CAD build for the part. Positions are in the model's coordinates, mm. A direction names the side the tool comes from. Coordinates: 2 decimals unless noted, no trailing zeros. Order: outer loops, then holes, each group sorted by start corner. A loop starts at its lowest first (then second) coordinate and runs counter-clockwise, first axis right, second up. Notation, with made-up numbers: (55.5, 8) - (109.5, 8) arc R26 cw to (109.5, 27) - close; hole circle Ø5 at (68, 0). An arc over 180 degrees is marked (long way). Write each question's results on one line, items separated by ' | '. Start each with the question number.
Q1. Wall check: probe 1 along Y at (x, z) = (2, -4); probe 2 along Z at (x, y) = (4, -3); probe 3 along Z at (x, y) = (-0.5, -10). Give the ranges that are in metal, low to high.
Q2. Band-saw the part on B-B, the plane x = 0. Write the cut outline in (y, z).
Q3. Which spindle directions (+Z, -Z, +X, -X, +Y, -Y) get a long thin tool onto all of the face, cutting with end or side? Do faces 5 (the flat face through (4.5, 0, -18)), 6 (the flat face through (-0.1, 7.934, -35.6)), 7 (the flat face through (0, 17.5, -3)). Say none if no direction does.
Q4. Band-saw the part on D-D, the plane y = -15.5. Write the cut outline in (x, z).
Q5. Pull direction Y, two halves, no side cores. Call faces 1 (the flat face through (0, 0, -35.181)), 2 (the flat face through (-0.063, 18.514, -32.62)), 3 (the flat face through (0, 0, -5.153)), 4 (the flat face through (0, 13, -36)): released by +Y, released by -Y, zero draft, split by the parting line, or undercut.
Q6. Band-saw the part on C-C, the plane y = 0.5. Write the cut outline in (x, z).
Q7. Pin check, flat tips, straight feed: P1, Ø2, axis at x = 1, y = -0.5, coming from the -Z side; P2, Ø2.5, axis at x = -0.5, y = -5, coming from the +Z side. Stop position of each tip, or through.
Q8. Band-saw the part on A-A, the plane z = -4.5. Write the cut outline in (x, y), then the cut area to 3 significant figures.
```python
from build123d import *

# Parameters (mm, degrees)
EXTRUDE_1_DEPTH      = 4.5
EXTRUDE_1_DEPTH_BACK = 4.5


with BuildPart() as part:
    # 草图1 → 凸台-拉伸1 (new, two sides: drawn at the far end of the back side and taken through both)
    with BuildSketch(Plane(origin=(0, 0, 0), x_dir=(0, 0, -1), z_dir=(1, 0, 0)).offset(-EXTRUDE_1_DEPTH_BACK)):
        Polygon((0, 17.5), (0, 19.5), (29.3330418, 19.5), (36, 17.5), (36, 7.934061775), (35.180915007, 7.934061775), (35.180915007, -7.934061775), (36, -7.934061775), (36, -17.5), (29.3330418, -19.5), (0, -19.5), (0, -17.5), (5.153343524, -17.5), (5.153343524, 17.5), align=None)
    extrude(amount=EXTRUDE_1_DEPTH + EXTRUDE_1_DEPTH_BACK)


solid = part.part
```
Results below:
1) probe 1: y = -19.5 to -17.5, 17.5 to 19.5 | probe 2: z = -35.18 to -5.15 | probe 3: z = -36 to -5.15
2) outline: (-19.5, -29.33) - (-17.5, -36) - (-7.93, -36) - (-7.93, -35.18) - (7.93, -35.18) - (7.93, -36) - (17.5, -36) - (19.5, -29.33) - (19.5, 0) - (17.5, 0) - (17.5, -5.15) - (-17.5, -5.15) - (-17.5, 0) - (-19.5, 0) - close
3) face 5: +Z, -Z, +X, +Y, -Y | face 6: -Z, +X, -X | face 7: +Z, +X, -X
4) outline: (-4.5, -36) - (4.5, -36) - (4.5, -5.15) - (-4.5, -5.15) - close
5) face 1: undercut | face 2: released by +Y | face 3: undercut | face 4: zero draft
6) outline: (-4.5, -35.18) - (4.5, -35.18) - (4.5, -5.15) - (-4.5, -5.15) - close
7) P1: stops at z = -35.18 | P2: stops at z = -5.15
8) outline: (-4.5, -19.5) - (4.5, -19.5) - (4.5, -17.5) - (-4.5, -17.5) - close; (-4.5, 17.5) - (4.5, 17.5) - (4.5, 19.5) - (-4.5, 19.5) - close | area: 36.0 mm²
